Geometry: final body of the model. Coordinates: model frame, mm. Face numbers are marked on the shaded views. A direction names the side the tool comes from. Coordinates: 2 decimals unless noted, no trailing zeros. Order: outer loops, then holes, each group sorted by start corner. A loop starts at its lowest first (then second) coordinate and runs counter-clockwise, first axis right, second up. Notation, with made-up numbers: (62.5, 67.5) -> (79.5, 67.5) arc R27 cw to (79.5, 88.5) -> close; hole circle Ø4 at (-13.5, -11.75). An arc over 180 degrees is marked (long way). Use one line per item in the form item = value.
```python
from build123d import *

# Parameters (mm, degrees)
SKETCH005_W     = 12
SKETCH005_H     = 13.2
SKETCH005_W_2   = 10.8
SKETCH005_H_2   = 12
PAD003_DEPTH    = 9.7
FILLET005_R     = 0.3
FILLET006_R     = 0.4
SKETCH006_W     = 1.85
SKETCH006_H     = 0.95
POCKET002_DEPTH = 0.6
FILLET007_R     = 0.13
SKETCH007_R     = 0.3
PAD004_DEPTH    = 1.3
FILLET008_R     = 0.1


with BuildPart() as part:
    # Sketch005 → Pad003 (new body)
    with BuildSketch(Plane.XY):
        with Locations((0, -1.1)):
            Rectangle(SKETCH005_W, SKETCH005_H)
        with Locations((0, -1.1)):
            Rectangle(SKETCH005_W_2, SKETCH005_H_2, mode=Mode.SUBTRACT)
    extrude(amount=PAD003_DEPTH)

    # Fillet005
    fillet005_edges = [part.edges().sort_by_distance(p)[0] for p in [
        (-6, 5.5, 4.85),
        (-6, -7.7, 4.85),
        (6, -7.7, 4.85),
        (6, 5.5, 4.85),
    ]]
    fillet(fillet005_edges, radius=FILLET005_R)

    # Fillet006
    fillet006_edges = [part.edges().sort_by_distance(p)[0] for p in [
        (-5.4, -7.1, 4.85),
        (-5.4, 4.9, 4.85),
        (5.4, -7.1, 4.85),
        (5.4, 4.9, 4.85),
    ]]
    fillet(fillet006_edges, radius=FILLET006_R)

    # Sketch006 (on Face10 of Fillet006) → Pocket002 (cut)
    with BuildSketch(Plane(origin=(0, 5.5, 0), x_dir=(-1, 0, 0), z_dir=(0, 1, 0))):
        with Locations((-3, 7.95)):
            Rectangle(SKETCH006_W, SKETCH006_H)
    pocket002 = extrude(amount=-POCKET002_DEPTH, mode=Mode.SUBTRACT)

    # Mirrored001: Pocket002 across Sketch006 V_Axis
    add(pocket002.mirror(Plane(origin=(0, 5.5, 0), x_dir=(0, 1, 0), z_dir=(-1, 0, 0))), mode=Mode.SUBTRACT)

    # Fillet007
    fillet007_edges = [part.edges().sort_by_distance(p)[0] for p in [
        (2.075, 5.2, 8.425),
        (2.075, 5.2, 7.475),
        (-3.925, 5.2, 7.475),
        (-3.925, 5.2, 8.425),
        (-2.075, 5.2, 8.425),
        (-2.075, 5.2, 7.475),
        (3.925, 5.2, 7.475),
        (3.925, 5.2, 8.425),
    ]]
    fillet(fillet007_edges, radius=FILLET007_R)

    # Sketch007 (on Face10 of Fillet007) → Pad004 (join)
    with BuildSketch(Plane(origin=(0, 0, 0), x_dir=(1, 0, 0), z_dir=(0, 0, -1))):
        with Locations((-5.586863, 7.286863)):
            Circle(SKETCH007_R)
        with Locations((5.586863, 7.286863)):
            Circle(SKETCH007_R)
        with Locations((-5.586863, -5.086863)):
            Circle(SKETCH007_R)
        with Locations((5.586863, -5.086863)):
            Circle(SKETCH007_R)
    extrude(amount=PAD004_DEPTH)

    # Fillet008
    fillet008_edges = [part.edges().sort_by_distance(p)[0] for p in [
        (5.286863, 5.086863, 0),
        (-5.886863, 5.086863, 0),
        (-5.886863, -7.286863, 0),
        (5.286863, -7.286863, 0),
    ]]
    fillet(fillet008_edges, radius=FILLET008_R)


solid = part.part
```
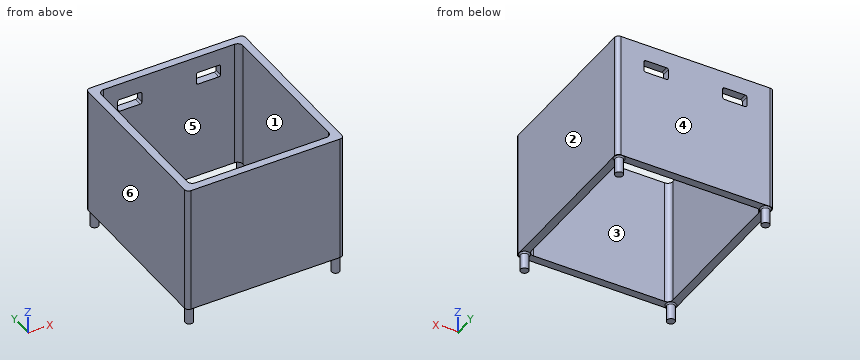
1) Section C-C, the plane x = -1. Output: boundary loops of the cut face in (y, z).
Results found:
outline = (-7.7, 0) -> (-7.1, 0) -> (-7.1, 9.7) -> (-7.7, 9.7) -> close; (4.9, 0) -> (5.5, 0) -> (5.5, 9.7) -> (4.9, 9.7) -> close
2) Section B-B, the plane y = -1. Output: boundary loops of the cut face in (x, z).
Results found:
outline = (-6, 0) -> (-5.4, 0) -> (-5.4, 9.7) -> (-6, 9.7) -> close; (5.4, 0) -> (6, 0) -> (6, 9.7) -> (5.4, 9.7) -> close
3) Section D-D, the plane z = 8. Output: boundary loops of the cut face in (x, y) (3 decimals).
Results found:
outline = (-6, -7.4) arc R0.3 ccw to (-5.7, -7.7) -> (5.7, -7.7) arc R0.3 ccw to (6, -7.4) -> (6, 5.2) arc R0.3 ccw to (5.7, 5.5) -> (3.925, 5.5) -> (3.925, 4.9) -> (5, 4.9) arc R0.4 cw to (5.4, 4.5) -> (5.4, -6.7) arc R0.4 cw to (5, -7.1) -> (-5, -7.1) arc R0.4 cw to (-5.4, -6.7) -> (-5.4, 4.5) arc R0.4 cw to (-5, 4.9) -> (-3.925, 4.9) -> (-3.925, 5.5) -> (-5.7, 5.5) arc R0.3 ccw to (-6, 5.2) -> close; (-2.075, 4.9) -> (2.075, 4.9) -> (2.075, 5.5) -> (-2.075, 5.5) -> close
4) Pull-direction query (X, two-part tool) for the marked faces 1, 2, 3 and 4; classes: released by +X, released by -X, zero draft, split by the parting line, or undercut.
Results found:
face_1 = undercut
face_2 = released by +X
face_3 = undercut
face_4 = zero draft
5) Access query for the marked faces 5 and 6. Directions: +Z, -Z, +X, -X, +Y, -Y. A direction counts if a zero-diameter tool reaches every point of the face in a straight line with its end or side. Return the directions, or none.
Results found:
face_5 = +Z, -Z
face_6 = +Z, -Z, -X, +Y, -Y
6) Contact query for flat-ended pins moving along their axis: P1, Ø3.5, axis at x = 0.5, y = -4, coming from the -Z side; P2, Ø0.5, axis at x = -3.5, y = 5.5, coming from the -Z side. Output: stop coordinate, or through.
Results found:
P1 = through
P2 = 0
7) Material intervals for probe 1 along Y at (x, z) = (0, 6.25); probe 2 along X at (y, z) = (0, 1); probe 3 along X at (y, z) = (-7, 4), sorted ascending. Write a range as from..to.
Results found:
probe_1 = -7.7..-7.1, 4.9..5.5
probe_2 = -6..-5.4, 5.4..6
probe_3 = -6..-5.26, 5.26..6
8) Section A-A, the plane x = -2.5. Output: boundary loops of the cut face in (y, z) (3 decimals), and give its area (3 significant figures).
Results found:
outline = (-7.7, 0) -> (-7.1, 0) -> (-7.1, 9.7) -> (-7.7, 9.7) -> close; (4.9, 0) -> (5.5, 0) -> (5.5, 7.475) -> (4.9, 7.475) -> close; (4.9, 8.425) -> (5.5, 8.425) -> (5.5, 9.7) -> (4.9, 9.7) -> close
area = 11.1 mm2
